The model under review builds one solid part; all positions refer to its coordinate system, in mm. A direction names the side the tool comes from. Round coordinates to 2 decimals unless told otherwise and drop trailing zeros. Write each loop counter-clockwise with the first axis right and the second up, starting at its lowest first coordinate (ties: lowest second). Pieces come first, ordered by that corner, then holes. Notation, with made-up numbers: M 89.5,21.5 L 110.5,21.5 A27 cw 110.5,41.5 Z; hole C 8,-36 d9. An arc over 180 degrees is marked long. Write item = value, one per line. Start each with the question number.
Item 1: Take a section at D-D, the plane y = 227. Give the boundary of the cut face in (x, z).
Item 2: Take a section at C-C, the plane y = 16.5. Give the boundary of the cut face in (x, z) (3 decimals).
Item 3: To check wall thickness, follow line 1 along Y through (x, z) = (0, 26.5); line 2 along Z through (x, y) = (25.5, 133.5); line 3 along X through (y, z) = (-25.5, 0.5). State the ranges of each line that lie inside material, in increasing order.
Item 4: For pin 1 Ø12 at (x, y) = (-21, 305) entering from -Z; pin 2 Ø10 at (y, z) = (397, 18) entering from -X; pin 3 Ø8 at (x, z) = (41.5, 32.5) entering from -Y, all flat-tipped, find the tip position at first contact; note any pin that passes through.
Item 5: Tool access review of faces 1 (the cylindrical face through (7.587, 465.832, -39.44)), 2 (the cylindrical face through (-1.539, -69.983, 29.58)): name each direction out of +Z, -Z, +X, -X, +Y, -Y from which nothing blocks a thin tool from reaching the whole face with its end or side.
Item 6: Take a section at A-A, the plane z = 20.5. Give the boundary of the cut face in (x, y).
Item 7: Take a section at B-B, the plane x = 0. Give the boundary of the cut face in (y, z).
from build123d import *

# Parameters (mm, degrees)
EXTRUDE_1_DEPTH     = 60
SKETCH_2_R          = 60
CUT_EXTRUDE_1_DEPTH = 60
SKETCH_3_R          = 35
EXTRUDE_2_DEPTH     = 80


with BuildPart() as part:
    # Эскиз1 → Бобышка-Вытянуть1 (new body)
    with BuildSketch(Plane.XY):
        with BuildLine():
            Line((-69.650872818, 6.982543641), (-70, 0))
            ThreePointArc((-70, 0), (0, -70), (70, 0))
            Line((70, 0), (69.650872818, 6.982543641))
            Line((69.650872818, 6.982543641), (45, 500))
            ThreePointArc((45, 500), (0, 545), (-45, 500))
            Line((-45, 500), (-69.650872818, 6.982543641))
        make_face()
    extrude(amount=EXTRUDE_1_DEPTH)

    # Эскиз2 → Вырез-Вытянуть1 (cut)
    with BuildSketch(Plane.XY.offset(60)):
        Circle(SKETCH_2_R)
    extrude(amount=-CUT_EXTRUDE_1_DEPTH, mode=Mode.SUBTRACT)

    # Эскиз3 → Бобышка-Вытянуть2 (add)
    with BuildSketch(Plane(origin=(0, 0, 0), x_dir=(-1, 0, 0), z_dir=(0, 0, -1))):
        with Locations((0, 500)):
            Circle(SKETCH_3_R)
    extrude(amount=EXTRUDE_2_DEPTH)


solid = part.part
Response values:
q1.outline = M -58.65,0 L 58.65,0 L 58.65,60 L -58.65,60 Z
q2.outline = M -69.175,0 L -57.687,0 L -57.687,60 L -69.175,60 Z; M 57.687,0 L 69.175,0 L 69.175,60 L 57.687,60 Z
q3.line_1 = -70 to -60, 60 to 545
q3.line_2 = 0 to 60
q3.line_3 = -65.19 to -54.31, 54.31 to 65.19
q4.pin_1 = 0
q4.pin_2 = -50.4
q4.pin_3 = -59.11
q5.face_1 = -Z
q5.face_2 = +Z, -Z, -Y
q6.outline = M -70,0 A70 ccw 70,0 L 45,500 A45 ccw -45,500 Z; hole C 0,0 d120
q7.outline = M -70,0 L -60,0 L -60,60 L -70,60 Z; M 60,0 L 465,0 L 465,-80 L 535,-80 L 535,0 L 545,0 L 545,60 L 60,60 Z
